Autodesk Inventor part; units mm, degrees
ref_plane "YZ Plane" through (0, 0, 0) normal (1, 0, 0) x (0, 1, 0)
ref_plane "XZ Plane" through (0, 0, 0) normal (0, 1, 0) x (-1, 0, 0)
ref_plane "XY Plane" through (0, 0, 0) normal (0, 0, 1) x (1, 0, 0)
sketch "Náčrt1" plane through (0, 0, 0) normal (0, 0, 1) x (1, 0, 0)
  line L0 (-21.25, 25) -> (21.25, 25)
  line L1 (21.25, 25) -> (21.25, -25)
  line L2 (21.25, -25) -> (-21.25, -25)
  line L3 (-21.25, -25) -> (-21.25, 25)
  line L4 (0, 35) -> (0, -35)
  line L5 (-29.75, 0) -> (29.75, 0)
  point P0 (0, 0)
  dimension "d0" = 50
  dimension "d1" = 42.5
extrude "Vysunutí1" add sketch "Náčrt1" along normal blind 3
sketch "Náčrt2" plane through (0, 0, 3) normal (0, 0, 1) x (1, 0, 0)
  line L0 (0, 35) -> (0, -35)
  line L1 (-29.75, 0) -> (29.75, 0)
  line L2 (21.25, -25) -> (21.25, 25)
  line L3 (21.25, 25) -> (-21.25, 25)
  line L4 (-21.25, 25) -> (-21.25, -25)
  line L5 (-21.25, -25) -> (21.25, -25)
  line L6 (-17.5, 21.5) -> (17.5, 21.5) construction
  line L7 (17.5, 21.5) -> (17.5, -21.5) construction
  line L8 (17.5, -21.5) -> (-17.5, -21.5) construction
  line L9 (-17.5, -21.5) -> (-17.5, 21.5) construction
  circle A0 centre (-14.75, 16) radius 1
  circle A1 centre (-14.75, -16) radius 1
  point P0 (0, 0)
  dimension "d4" = 35
  dimension "d5" = 43
  dimension "d6" = 2
  dimension "d9" = 16
  dimension "d10" = 36
extrude "Vysunutí2" add sketch "Náčrt2" along normal blind 3 contours A0 | A1
sketch "Náčrt3" plane through (0, 0, 3) normal (0, 0, 1) x (1, 0, 0)
  circle A0 centre (-14.75, -16) radius 1
  circle A1 centre (-14.75, 16) radius 1
  line L0 (21.25, -25) -> (21.25, 25)
  line L1 (21.25, 25) -> (-21.25, 25)
  line L2 (-21.25, 25) -> (-21.25, -25)
  line L3 (-21.25, -25) -> (21.25, -25)
  line L4 (0, 35) -> (0, -35)
  line L5 (-29.75, 0) -> (29.75, 0)
  line L6 (-23.75, 27.5) -> (23.75, 27.5)
  line L7 (23.75, 27.5) -> (23.75, -27.5)
  line L8 (23.75, -27.5) -> (-23.75, -27.5)
  line L9 (-23.75, -27.5) -> (-23.75, 27.5)
  line L10 (-21.25, 25) -> (21.25, 25)
  line L11 (21.25, 25) -> (21.25, -25)
  line L12 (21.25, -25) -> (-21.25, -25)
  line L13 (-21.25, -25) -> (-21.25, 25)
  point P0 (0, 0)
  dimension "d13" = 2.5
extrude "Vysunutí3" add sketch "Náčrt3" along normal blind 25 and the other way blind 3 contours L0 L5 L7 L8 L4 L3 | L0 L1 L4 L6 L7 L5 | L4 L8 L9 L5 L2 L3 | L1 L2 L5 L9 L6 L4
sketch "Náčrt4" plane through (23.75, -27.5, 28) normal (1, 0, 0) x (0, 0, -1)
  line L0 (13, 34) -> (21, 34)
  line L1 (21, 34) -> (21, 49)
  line L2 (21, 49) -> (13, 49)
  line L3 (13, 49) -> (13, 34)
  line L4 (0, 55) -> (28, 55)
  line L5 (0, 0) -> (0, 55)
  line L6 (28, 0) -> (0, 0)
  line L7 (28, 55) -> (28, 0)
  line L8 (-6.6, 27.5) -> (39.6, 27.5)
  line L9 (28, -11) -> (28, 66)
  line L10 (25, 2.5) -> (25, 52.5)
  line L11 (0, 52.5) -> (25, 52.5)
  point P0 (28, 27.5)
  dimension "d18" = 15
  dimension "d19" = 8
  dimension "d20" = 7
  dimension "d21" = 6
extrude "Vysunutí4" cut sketch "Náčrt4" against normal up to surface (2.5 mm away) contours L3 L2 L1 L0
sketch "Náčrt5" plane through (-23.75, -27.5, 28) normal (0, -1, 0) x (1, 0, 0)
  line L0 (47.5, -28) -> (47.5, 0)
  line L1 (0, 0) -> (47.5, 0)
  line L2 (0, -28) -> (0, 0)
  line L3 (47.5, -28) -> (0, -28)
  line L4 (23.75, 99) -> (23.75, -55)
  line L5 (-9.5, -28) -> (57, -28)
  line L6 (31.25, -28) -> (16.25, -28)
  line L7 (16.25, -28) -> (16.25, 77)
  line L8 (16.25, 77) -> (31.25, 77)
  line L9 (31.25, 77) -> (31.25, -28)
  point P0 (23.75, -28)
  point P1 (31.25, -28)
  dimension "d24" = 15
  dimension "d25" = 77
extrude "Vysunutí5" add sketch "Náčrt5" along normal blind 5 contours L3 L4 L1 L9 | L1 L4 L8 L9 | L3 L7 L1 L4 | L1 L7 L8 L4
sketch "Náčrt6" plane through (-23.75, -32.5, 28) normal (0, -1, 0) x (1, 0, 0)
  line L0 (16.25, 77) -> (16.25, -28)
  line L1 (16.25, -28) -> (31.25, -28)
  line L2 (31.25, -28) -> (31.25, 77)
  line L3 (31.25, 77) -> (16.25, 77)
  line L4 (23.75, 99) -> (23.75, -55)
  line L5 (-9.5, -28) -> (57, -28)
  point P0 (23.75, -28)
  point P1 (23.75, 62)
  dimension "d28" = 15
hole "Díra1" at (0, -32.5, 90) direction (0, 1, 0) diameter 6.6 end through all
chamfer "Zkosení1" distance 1 angle 45 4 edges at (-7.5, -32.5, 52.5) (7.5, -32.5, 52.5) (0, -32.5, 105) (0, -32.5, 0)
fillet "Zaoblení1" radius 2 4 edges at (-23.75, -27.5, 14) (23.75, -27.5, 14) (23.75, 27.5, 14) (-23.75, 27.5, 14)
properties part number "a4988_box_3D tisk"
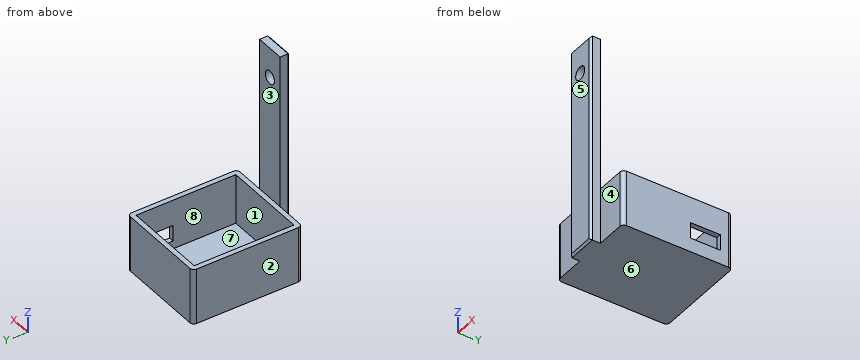
Source: CAD feature listing. Evaluate the final solid. Frame: model axes, mm. Face numbers are marked on the shaded views. A direction names the side the tool comes from. Round coordinates to 2 decimals unless told otherwise and drop trailing zeros. Loops run counter-clockwise (first coordinate to the right, second up) from the corner with the lowest first, then second, coordinate; pieces in that order, holes last. Notation, with made-up numbers: M 20,62.5 L 34,62.5 A8 cw 34,74.5 Z; hole C 76.5,74.5 d4. An arc over 180 degrees is marked long. Use a Markdown table: item, result. Add a question column.
1. Section query C-C on x = 0. Return the cut outline in (y, z).
2. Section query D-D on x = 18. Return the cut outline in (y, z).
3. Reachability of the marked faces 1, 2, 3 and 4 from +Z, -Z, +X, -X, +Y, -Y: full face, straight path, thin tool, end or side. Return the list, or none.
4. Section query A-A on y = 9. Return the cut outline in (x, z).
5. Contact query for flat-ended pins moving along their axis: P1, Ø3, axis at x = 22.5, y = 14, coming from the +Z side; P2, Ø12, axis at x = 1, z = 65.5, coming from the +Y side; P3, Ø13, axis at x = 9, y = -4, coming from the +Z side. Output: stop coordinate, or through.
6. Mould query, pull axis Y, two halves, no side actions, for the marked faces 5, 6, 7 and 8. Classes: pulls with the +Y half, pulls with the -Y half, needs draft (parallel to the pull), parting line crosses it, or undercut.
7. Line query: line 1 (Z direction, x = 0, y = -30.4); line 2 (X direction, y = -31.35, z = 90); line 3 (X direction, y = -17, z = 10.5). Output: solid intervals per line, ascending.
8. Section query B-B on z = 90. Return the cut outline in (x, y).
Reported:
| question | item | result |
|---|---|---|
| 1 | outline | M -32.5,1 L -31.5,0 L 27.5,0 L 27.5,28 L 25,28 L 25,3 L -25,3 L -25,28 L -27.5,28 L -27.5,86.7 L -32.5,86.7 Z; M -32.5,93.3 L -27.5,93.3 L -27.5,105 L -31.5,105 L -32.5,104 Z |
| 2 | outline | M -27.5,0 L 27.5,0 L 27.5,28 L 25,28 L 25,3 L -25,3 L -25,28 L -27.5,28 Z |
| 3 | face 1 | +Z |
| 3 | face 2 | +Z, -Z, -X, +Y, -Y |
| 3 | face 3 | +Z, +X, -X, +Y |
| 3 | face 4 | +Z, -Z, +X, -Y |
| 4 | outline | M -23.75,0 L 23.75,0 L 23.75,7 L 21.25,7 L 21.25,3 L -21.25,3 L -21.25,28 L -23.75,28 Z; M 21.25,15 L 23.75,15 L 23.75,28 L 21.25,28 Z |
| 5 | P1 | stops at z = 28 |
| 5 | P2 | stops at y = -27.5 |
| 5 | P3 | stops at z = 3 |
| 6 | face 5 | pulls with the -Y half |
| 6 | face 6 | needs draft |
| 6 | face 7 | undercut |
| 6 | face 8 | undercut |
| 7 | line 1 | z = 0 to 86.7, 93.3 to 105 |
| 7 | line 2 | x = -7.5 to -3.3, 3.3 to 7.5 |
| 7 | line 3 | x = -23.75 to -21.25, 21.25 to 23.75 |
| 8 | outline | M -7.5,-31.5 L -6.5,-32.5 L -3.3,-32.5 L -3.3,-27.5 L -7.5,-27.5 Z; M 3.3,-32.5 L 6.5,-32.5 L 7.5,-31.5 L 7.5,-27.5 L 3.3,-27.5 Z |
